Geometry check sheet. Reference: the model listing, model coordinates, mm. Face numbers are marked on the shaded views. A direction names the side the tool comes from. Round coordinates to 2 decimals unless told otherwise and drop trailing zeros. Order: outer loops, then holes, each group sorted by start corner. A loop starts at its lowest first (then second) coordinate and runs counter-clockwise, first axis right, second up. Notation, with made-up numbers: (29.5, 19.25) - (33.5, 19.25) arc R31 ccw to (33.5, 53.25) - close; hole circle Ø11 at (82.5, 26). An arc over 180 degrees is marked (long way). Return JSON: item names as keys, results as strings. Group by question number.
Q1. Tool access check on the marked faces 1 and 2. Record the directions out of +Z, -Z, +X, -X, +Y, -Y that give a thin tool (end or side, any length) a straight path to the whole face; none if there is none.
Q2. Material ranges on line 1 along Y through (x, z) = (4.5, 2.25); line 2 along Z through (x, y) = (0, -3); line 3 along Y through (x, z) = (5.25, 12.25), recorded low to high.
Q3. Gauge pin test, flat ends, axial feed: pin 1 Ø2 at (x, y) = (-5, 1.5) entering from +Z; pin 2 Ø2 at (y, z) = (-3.5, 4) entering from +X; pin 3 Ø5 at (y, z) = (2.5, 20) entering from -X. Record the tip position at first contact, or that the pin passes through.
Q4. Sectioned sample at A-A, the plane z = 15.5. Record the cut outline in (x, y).
```python
from build123d import *

# Parameters (mm, degrees)
SKETCH1_R           = 5
BOSS_EXTRUDE1_DEPTH = 15
SKETCH1_3_R         = 2.6
BOSS_EXTRUDE2_DEPTH = 25
BOSS_EXTRUDE3_DEPTH = 15


with BuildPart() as part:
    # Sketch1 → Boss-Extrude1 (new body)
    with BuildSketch(Plane.XY):
        Circle(SKETCH1_R)
    extrude(amount=BOSS_EXTRUDE1_DEPTH)

    # Sketch1<3> → Boss-Extrude2 (add)
    with BuildSketch(Plane.XY):
        Circle(SKETCH1_3_R)
    extrude(amount=BOSS_EXTRUDE2_DEPTH)

    # Sketch2 → Boss-Extrude3 (add)
    with BuildSketch(Plane(origin=(0, 0, 0), x_dir=(-1, 0, 0), z_dir=(0, 0, -1))):
        with BuildLine():
            Line((0.436151452, 5.994353336), (1.130162855, 5.902985001))
            Line((1.130162855, 5.902985001), (1.294095226, 4.829629131))
            ThreePointArc((1.294095226, 4.829629131), (0.652630961, 4.957224307), (0, 5))
            Line((0, 5), (0.436151452, 5.994353336))
        make_face()
        with BuildLine():
            Line((2.460037888, 5.483677014), (3.080945471, 5.160452984))
            Line((3.080945471, 5.160452984), (2.867882182, 4.095760221))
            ThreePointArc((2.867882182, 4.095760221), (2.308743066, 4.435054166), (1.710100717, 4.698463104))
            Line((1.710100717, 4.698463104), (2.460037888, 5.483677014))
        make_face()
        with BuildLine():
            Line((4.187207448, 4.311588314), (4.660120594, 3.795494178))
            Line((4.660120594, 3.795494178), (4.095760221, 2.867882182))
            ThreePointArc((4.095760221, 2.867882182), (3.686386684, 3.377951038), (3.213938048, 3.830222216))
            Line((3.213938048, 3.830222216), (4.187207448, 4.311588314))
        make_face()
        with BuildLine():
            Line((5.409337994, 2.619458431), (5.677216396, 1.972742758))
            Line((5.677216396, 1.972742758), (4.829629131, 1.294095226))
            ThreePointArc((4.829629131, 1.294095226), (4.619397663, 1.913417162), (4.330127019, 2.5))
            Line((4.330127019, 2.5), (5.409337994, 2.619458431))
        make_face()
        with BuildLine():
            Line((5.979022544, 0.611383202), (6.009556115, -0.087950553))
            Line((6.009556115, -0.087950553), (4.98097349, -0.435778714))
            ThreePointArc((4.98097349, -0.435778714), (4.995241108, 0.218096937), (4.924038765, 0.868240888))
            Line((4.924038765, 0.868240888), (5.979022544, 0.611383202))
        make_face()
        with BuildLine():
            Line((5.827548734, -1.470433864), (5.617054675, -2.13803573))
            Line((5.617054675, -2.13803573), (4.531538935, -2.113091309))
            ThreePointArc((4.531538935, -2.113091309), (4.768584754, -1.503528998), (4.924038765, -0.868240888))
            Line((4.924038765, -0.868240888), (5.827548734, -1.470433864))
        make_face()
        with BuildLine():
            Line((4.973186542, -3.374894905), (4.547053542, -3.930242243))
            Line((4.547053542, -3.930242243), (3.535533906, -3.535533906))
            ThreePointArc((3.535533906, -3.535533906), (3.966766701, -3.043807145), (4.330127019, -2.5))
            Line((4.330127019, -2.5), (4.973186542, -3.374894905))
        make_face()
        with BuildLine():
            Line((3.518984656, -4.872293812), (2.928610644, -5.248403538))
            Line((2.928610644, -5.248403538), (2.113091309, -4.531538935))
            ThreePointArc((2.113091309, -4.531538935), (2.686498042, -4.216957229), (3.213938048, -3.830222216))
            Line((3.213938048, -3.830222216), (3.518984656, -4.872293812))
        make_face()
        with BuildLine():
            Line((1.640341286, -5.782022178), (0.956934081, -5.933529908))
            Line((0.956934081, -5.933529908), (0.435778714, -4.98097349))
            ThreePointArc((0.435778714, -4.98097349), (1.08219807, -4.881480036), (1.710100717, -4.698463104))
            Line((1.710100717, -4.698463104), (1.640341286, -5.782022178))
        make_face()
        with BuildLine():
            Line((-0.436151452, -5.994353336), (-1.130162855, -5.902985001))
            Line((-1.130162855, -5.902985001), (-1.294095226, -4.829629131))
            ThreePointArc((-1.294095226, -4.829629131), (-0.652630961, -4.957224307), (0, -5))
            Line((0, -5), (-0.436151452, -5.994353336))
        make_face()
        with BuildLine():
            Line((-2.460037888, -5.483677014), (-3.080945471, -5.160452984))
            Line((-3.080945471, -5.160452984), (-2.867882182, -4.095760221))
            ThreePointArc((-2.867882182, -4.095760221), (-2.308743066, -4.435054166), (-1.710100717, -4.698463104))
            Line((-1.710100717, -4.698463104), (-2.460037888, -5.483677014))
        make_face()
        with BuildLine():
            Line((-4.187207448, -4.311588314), (-4.660120594, -3.795494178))
            Line((-4.660120594, -3.795494178), (-4.095760221, -2.867882182))
            ThreePointArc((-4.095760221, -2.867882182), (-3.686386684, -3.377951038), (-3.213938048, -3.830222216))
            Line((-3.213938048, -3.830222216), (-4.187207448, -4.311588314))
        make_face()
        with BuildLine():
            Line((-5.409337994, -2.619458431), (-5.677216396, -1.972742758))
            Line((-5.677216396, -1.972742758), (-4.829629131, -1.294095226))
            ThreePointArc((-4.829629131, -1.294095226), (-4.619397663, -1.913417162), (-4.330127019, -2.5))
            Line((-4.330127019, -2.5), (-5.409337994, -2.619458431))
        make_face()
        with BuildLine():
            Line((-5.979022544, -0.611383202), (-6.009556115, 0.087950553))
            Line((-6.009556115, 0.087950553), (-4.98097349, 0.435778714))
            ThreePointArc((-4.98097349, 0.435778714), (-4.995241108, -0.218096937), (-4.924038765, -0.868240888))
            Line((-4.924038765, -0.868240888), (-5.979022544, -0.611383202))
        make_face()
        with BuildLine():
            Line((-5.827548734, 1.470433864), (-5.617054675, 2.13803573))
            Line((-5.617054675, 2.13803573), (-4.531538935, 2.113091309))
            ThreePointArc((-4.531538935, 2.113091309), (-4.768584754, 1.503528998), (-4.924038765, 0.868240888))
            Line((-4.924038765, 0.868240888), (-5.827548734, 1.470433864))
        make_face()
        with BuildLine():
            Line((-4.973186542, 3.374894905), (-4.547053542, 3.930242243))
            Line((-4.547053542, 3.930242243), (-3.535533906, 3.535533906))
            ThreePointArc((-3.535533906, 3.535533906), (-3.966766701, 3.043807145), (-4.330127019, 2.5))
            Line((-4.330127019, 2.5), (-4.973186542, 3.374894905))
        make_face()
        with BuildLine():
            Line((-3.518984656, 4.872293812), (-2.928610644, 5.248403538))
            Line((-2.928610644, 5.248403538), (-2.113091309, 4.531538935))
            ThreePointArc((-2.113091309, 4.531538935), (-2.686498042, 4.216957229), (-3.213938048, 3.830222216))
            Line((-3.213938048, 3.830222216), (-3.518984656, 4.872293812))
        make_face()
        with BuildLine():
            Line((-1.640341286, 5.782022178), (-0.956934081, 5.933529908))
            Line((-0.956934081, 5.933529908), (-0.435778714, 4.98097349))
            ThreePointArc((-0.435778714, 4.98097349), (-1.08219807, 4.881480036), (-1.710100717, 4.698463104))
            Line((-1.710100717, 4.698463104), (-1.640341286, 5.782022178))
        make_face()
    extrude(amount=-BOSS_EXTRUDE3_DEPTH)


solid = part.part
```
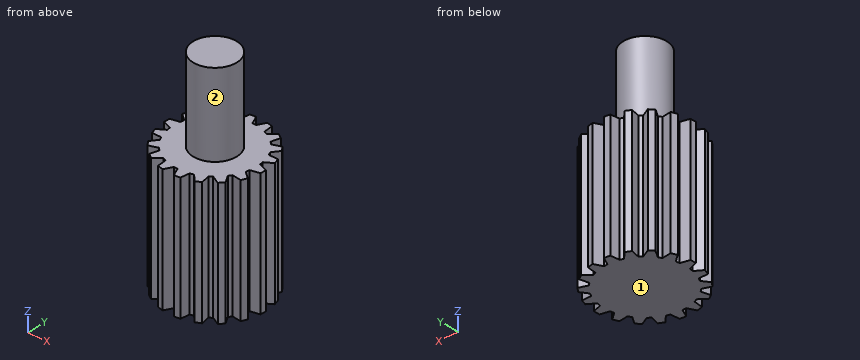
Reply:
{
 "1": {"face 1": "-Z, +X, -X, +Y, -Y", "face 2": "+Z"},
 "2": {"line 1": "-3.97 to -3.53, -2.52 to 2.18, 2.73 to 3.91", "line 2": "0 to 15", "line 3": "-2.6 to -1.63, -0.79 to 0.34, 1.09 to 2.13"},
 "3": {"pin 1": "z = 15", "pin 2": "x = 5.46", "pin 3": "x = -2.6"},
 "4": {"outline": "circle Ø5.2 at (0, 0)"}
}
